from build123d import *

# Parameters (mm, degrees)
F0_R     = 3.429
F0_R_2   = 2.159
F1_DEPTH = 8.509
F2_DEPTH = 6.35


with BuildPart() as f1:
    # F0 (on Top) → F1 (new body)
    with BuildSketch(Plane.XY):
        with BuildLine():
            Line((0, 11.938), (0, 13.2588))
            Line((0, 13.2588), (-6.9088, 13.2588))
            ThreePointArc((-6.9088, 13.2588), (-11.398928, 11.398928), (-13.2588, 6.9088))
            Line((-13.2588, 6.9088), (-13.2588, -6.9088))
            ThreePointArc((-13.2588, -6.9088), (-11.398928, -11.398928), (-6.9088, -13.2588))
            Line((-6.9088, -13.2588), (0, -13.2588))
            Line((0, -13.2588), (0, -11.938))
            ThreePointArc((0, -11.938), (-2.159, -9.779), (0, -7.62))
            Line((0, -7.62), (0, -2.159))
            ThreePointArc((0, -2.159), (-2.159, 0), (0, 2.159))
            Line((0, 2.159), (0, 7.62))
            ThreePointArc((0, 7.62), (-2.159, 9.779), (0, 11.938))
        make_face()
        with Locations((-6.9088, -6.9088)):
            Circle(F0_R, mode=Mode.SUBTRACT)
        with Locations((-9.779, 0)):
            Circle(F0_R_2, mode=Mode.SUBTRACT)
        with Locations((-6.9088, 6.9088)):
            Circle(F0_R, mode=Mode.SUBTRACT)
        with BuildLine():
            ThreePointArc((13.2588, 6.9088), (11.398928, 11.398928), (6.9088, 13.2588))
            Line((6.9088, 13.2588), (0, 13.2588))
            Line((0, 13.2588), (0, 11.938))
            ThreePointArc((0, 11.938), (1.526644, 11.305644), (2.159, 9.779))
            ThreePointArc((2.159, 9.779), (1.526644, 8.252356), (0, 7.62))
            Line((0, 7.62), (0, 2.159))
            ThreePointArc((0, 2.159), (1.526644, 1.526644), (2.159, 0))
            ThreePointArc((2.159, 0), (1.526644, -1.526644), (0, -2.159))
            Line((0, -2.159), (0, -7.62))
            ThreePointArc((0, -7.62), (1.526644, -8.252356), (2.159, -9.779))
            ThreePointArc((2.159, -9.779), (1.526644, -11.305644), (0, -11.938))
            Line((0, -11.938), (0, -13.2588))
            Line((0, -13.2588), (6.9088, -13.2588))
            ThreePointArc((6.9088, -13.2588), (11.398928, -11.398928), (13.2588, -6.9088))
            Line((13.2588, -6.9088), (13.2588, 6.9088))
        make_face()
        with Locations((6.9088, -6.9088)):
            Circle(F0_R, mode=Mode.SUBTRACT)
        with Locations((9.779, 0)):
            Circle(F0_R_2, mode=Mode.SUBTRACT)
        with Locations((6.9088, 6.9088)):
            Circle(F0_R, mode=Mode.SUBTRACT)
        with Locations((-6.9088, 6.9088)):
            Circle(F0_R)
        with Locations((-6.9088, 6.9088)):
            Circle(F0_R_2, mode=Mode.SUBTRACT)
        with Locations((-6.9088, -6.9088)):
            Circle(F0_R)
        with Locations((-6.9088, -6.9088)):
            Circle(F0_R_2, mode=Mode.SUBTRACT)
        with Locations((6.9088, -6.9088)):
            Circle(F0_R)
        with Locations((6.9088, -6.9088)):
            Circle(F0_R_2, mode=Mode.SUBTRACT)
        with Locations((6.9088, 6.9088)):
            Circle(F0_R)
        with Locations((6.9088, 6.9088)):
            Circle(F0_R_2, mode=Mode.SUBTRACT)
    extrude(amount=F1_DEPTH)

    # F0 (on Top) → F2 (cut)
    with BuildSketch(Plane.XY):
        with Locations((-6.9088, -6.9088)):
            Circle(F0_R)
        with Locations((-6.9088, -6.9088)):
            Circle(F0_R_2, mode=Mode.SUBTRACT)
        with Locations((6.9088, -6.9088)):
            Circle(F0_R)
        with Locations((6.9088, -6.9088)):
            Circle(F0_R_2, mode=Mode.SUBTRACT)
        with Locations((6.9088, 6.9088)):
            Circle(F0_R)
        with Locations((6.9088, 6.9088)):
            Circle(F0_R_2, mode=Mode.SUBTRACT)
        with Locations((-6.9088, 6.9088)):
            Circle(F0_R)
        with Locations((-6.9088, 6.9088)):
            Circle(F0_R_2, mode=Mode.SUBTRACT)
    extrude(amount=F2_DEPTH, mode=Mode.SUBTRACT)


solid = f1.part
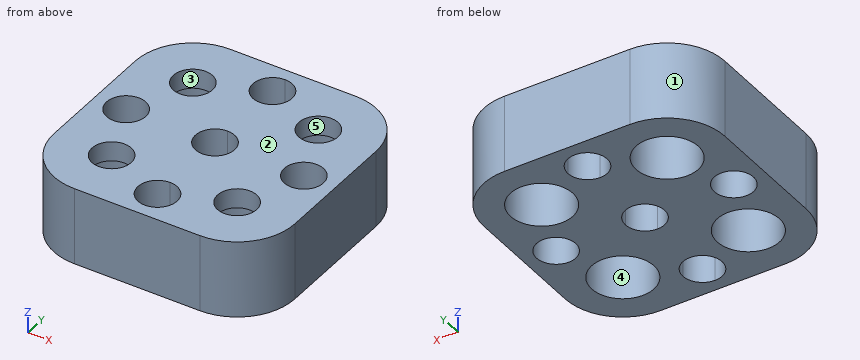
Input: part model. Units: mm. Frame: model coordinates. Face numbers are marked on the shaded views. A direction names the side the tool comes from. Coordinates: 2 decimals unless noted, no trailing zeros. Loops run counter-clockwise (first coordinate to the right, second up) from the corner with the lowest first, then second, coordinate; pieces in that order, holes last.
Q1. Cut plane B-B (y = 8.5). Output: boundary loops of the cut face in (x, z).
Q2. Cut plane A-A (x = -11.25). Output: boundary loops of the cut face in (y, z).
Q3. Cut plane C-C (x = 6). Output: boundary loops of the cut face in (y, z).
Q4. Contact query for a flat-ended pin moving along its axis: pin 1 (2.5 mm diameter, centred on x = -9.779, y = 0, fed in from -Z). Output: stop coordinate, or through.
Q5. Material intervals for line 1 (Y direction, x = 7, z = 3.5); line 2 (Y direction, x = 7, z = 6.75); line 3 (X direction, y = 8.5, z = 4.75), sorted ascending.
Q6. Set-up query: the marked faces 4 and 5. Return all of +Z, -Z, +X, -X, +Y, -Y with unobstructed straight access to the full face (end or side cutting, diameter ignored); none if empty.
Q7. Draft query along X for the marked faces 1, 2 and 3. Return one class per face: +X half, -X half, draft (parallel to the pull), parting line (faces both ways), or undercut.
Q8. Cut plane D-D (z = 5.25). Give the number of separate pieces and of enclosed holes in the cut face, then the cut area to 3 significant figures.
Working result:
1. outline: (-13.06, 0) - (-9.95, 0) - (-9.95, 6.35) - (-8.37, 6.35) - (-8.37, 8.51) - (-13.06, 8.51) - close; (-5.45, 6.35) - (-3.87, 6.35) - (-3.87, 0) - (-1.74, 0) - (-1.74, 8.51) - (-5.45, 8.51) - close; (1.74, 0) - (3.87, 0) - (3.87, 6.35) - (5.45, 6.35) - (5.45, 8.51) - (1.74, 8.51) - close; (8.37, 6.35) - (9.95, 6.35) - (9.95, 0) - (13.06, 0) - (13.06, 8.51) - (8.37, 8.51) - close
2. outline: (-11.54, 0) - (-1.58, 0) - (-1.58, 8.51) - (-11.54, 8.51) - close; (1.58, 0) - (11.54, 0) - (11.54, 8.51) - (1.58, 8.51) - close
3. outline: (-13.26, 0) - (-10.22, 0) - (-10.22, 6.35) - (-8.87, 6.35) - (-8.87, 8.51) - (-13.26, 8.51) - close; (-4.95, 6.35) - (-3.6, 6.35) - (-3.6, 0) - (3.6, 0) - (3.6, 6.35) - (4.95, 6.35) - (4.95, 8.51) - (-4.95, 8.51) - close; (8.87, 6.35) - (10.22, 6.35) - (10.22, 0) - (13.26, 0) - (13.26, 8.51) - (8.87, 8.51) - close
4. pin 1: passes through
5. line 1: y = -13.26 to -10.34, -3.48 to 3.48, 10.34 to 13.26
5. line 2: y = -13.26 to -9.07, -4.75 to 4.75, 9.07 to 13.26
5. line 3: x = -13.06 to -9.95, -3.87 to -1.74, 1.74 to 3.87, 9.95 to 13.06
6. face 4: -Z
6. face 5: +Z, -Z
7. face 1: -X half
7. face 2: draft
7. face 3: undercut
8. separate pieces: 1
8. enclosed holes: 9
8. area: 448 mm2
